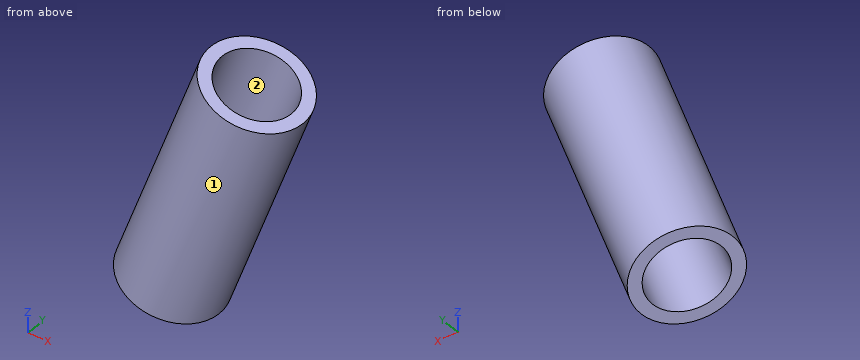
```python
from build123d import *

# Parameters (mm, degrees)
CYLINDER001_R      = 3
CYLINDER001_DEPTH  = 20
CYLINDER_R         = 4
CYLINDER_DEPTH     = 20
CUT001_PITCH_ANGLE = 20


with BuildPart() as tubeinside:
    # Cylinder001 → Cylinder001 (new body)
    with BuildSketch(Plane.XY):
        Circle(CYLINDER001_R)
    extrude(amount=CYLINDER001_DEPTH)


with BuildPart() as tube:
    # Cylinder → Cylinder (new body)
    with BuildSketch(Plane.XY):
        Circle(CYLINDER_R)
    extrude(amount=CYLINDER_DEPTH)

    # Cut001: cut TubeInside
    add(tubeinside.part, mode=Mode.SUBTRACT)


with BuildPart() as tube_1:
    # Cut001 pitch: moved
    add(tube.part.rotate(Axis((0, 0, 0), (0, 1, 0)), CUT001_PITCH_ANGLE))


with BuildPart() as tube_2:
    # Cut001 placement: moved
    add(tube_1.part)


solid = tube_2.part
```
Check sheet for the modelled part. Datum: model origin and axes. Units: mm. Face numbers are marked on the shaded views. Give positions to 0.01 mm unless a question says otherwise; leave off trailing zeros. Order: outer loops, then holes, each group sorted by start corner. A loop starts at its lowest first (then second) coordinate and runs counter-clockwise, first axis right, second up. Notation, with made-up numbers: M 71,87.25 L 75,87.25 A20 ccw 75,94.25 Z; hole C -31,78 d9. An arc over 180 degrees is marked long. Answer in a Markdown table with one row per item. Add a question column.
Q1. Sectioned sample at A-A, the plane y = -1.25. Record the boundary of the cut face in (x, z).
Q2. Release check for a two-part mould opening along Z. For the marked faces 1 and 2 record: released by +Z, released by -Z, zero draft, split by the parting line, or undercut.
Q3. Sectioned sample at B-B, the plane y = -2.5. Record the boundary of the cut face in (x, z), and give its area (3 significant figures).
Q4. Gauge pin test, flat ends, axial feed: pin 1 Ø3 at (x, z) = (-0.5, 12) entering from +Y; pin 2 Ø5 at (x, z) = (-0.5, 7) entering from +Y; pin 3 Ø3 at (x, z) = (3.5, 2.5) entering from -Y. Record the tip position at first contact, or that the pin passes through.
Q5. Thickness scan on L1, parallel to Y at x = 6, z = 17; L2, parallel to X at y = 1.5, z = 10.5; L3, parallel to Y at x = -0.5, z = 3.25. Record the ranges inside material, lowest first.
Verdict:
| question | item | result |
|---|---|---|
| 1 | outline | M -3.57,1.3 L -2.56,0.93 L 4.28,19.73 L 3.27,20.09 Z; M 2.56,-0.93 L 3.57,-1.3 L 10.41,17.49 L 9.4,17.86 Z |
| 2 | face 1 | split by the parting line |
| 2 | face 2 | undercut |
| 3 | outline | M -2.93,1.07 L -1.56,0.57 L 5.28,19.36 L 3.91,19.86 Z; M 1.56,-0.57 L 2.93,-1.07 L 9.77,17.73 L 8.4,18.23 Z |
| 3 | area | 58.6 mm² |
| 4 | pin 1 | y = 2.56 |
| 4 | pin 2 | y = 3.98 |
| 4 | pin 3 | y = -3.89 |
| 5 | L1 | -4 to -2.99, 2.99 to 4 |
| 5 | L2 | -0.12 to 1.06, 6.59 to 7.77 |
| 5 | L3 | -3.67 to -2.55, 2.55 to 3.67 |
